Part model, mm, in its own coordinate system. A direction names the side the tool comes from. Coordinates: 2 decimals unless noted, no trailing zeros. Write each loop counter-clockwise with the first axis right and the second up, starting at its lowest first coordinate (ties: lowest second). Pieces come first, ordered by that corner, then holes. Notation, with made-up numbers: (-17.75, -17) - (19.25, -17) arc R31 ccw to (19.25, 14) - close; hole circle Ø6 at (83.25, -27.75). An arc over 180 degrees is marked (long way). Use a Markdown table: item, result.
```python
from build123d import *

# Parameters (mm, degrees)
SKETCH1_W             = 4.084
SKETCH1_H             = 6.24
EXTRUDE1_DEPTH        = 7
SKETCH6_W             = 6.834
SKETCH6_H             = 16.75
EXTRUDE2_DEPTH        = 5.23
F_4_CLEARANCE_HOLE1_D = 3.2
SKETCH3_R             = 1.25
CUT_EXTRUDE1_DEPTH    = 7.24
SKETCH7_W             = 0.217
SKETCH7_H             = 16.75
EXTRUDE3_DEPTH        = 6.23


with BuildPart() as part:
    # Sketch1 → Extrude1 (new body, symmetric)
    with BuildSketch(Plane.XY):
        Rectangle(SKETCH1_W, SKETCH1_H)
    extrude(amount=EXTRUDE1_DEPTH, both=True)

    # Sketch6 → Extrude2 (add)
    with BuildSketch(Plane(origin=(0, 3.12, 0), x_dir=(1, 0, 0), z_dir=(0, 1, 0))):
        Rectangle(SKETCH6_W, SKETCH6_H)
    extrude(amount=-EXTRUDE2_DEPTH)

    # 4 Clearance Hole1 (through all)
    with Locations(Plane(origin=(0.396685659, -3.12, 2.776888518), x_dir=(1, 0, 0), z_dir=(0, -1, 0))):
        with Locations((-0.396685659, -2.776888518)):
            Hole(F_4_CLEARANCE_HOLE1_D / 2)

    # Sketch3 → Cut-Extrude1 (cut, through all)
    with BuildSketch(Plane(origin=(0, -3.12, 0), x_dir=(-1, 0, 0), z_dir=(0, -1, 0))):
        with Locations(Location((0, -5, 0), (0, 0, 180))):  # turned: the seam where the file's is
            Circle(SKETCH3_R)
        with Locations((0, 5)):
            Circle(SKETCH3_R)
    extrude(amount=-CUT_EXTRUDE1_DEPTH, mode=Mode.SUBTRACT)

    # Sketch7 → Extrude3 (cut, through all)
    with BuildSketch(Plane.XZ.offset(2.11)):
        with Locations((3.3085, 0)):
            Rectangle(SKETCH7_W, SKETCH7_H)
    extrude3 = extrude(amount=-EXTRUDE3_DEPTH, mode=Mode.SUBTRACT)

    # Mirror1: Extrude3 across plane
    add(extrude3.mirror(Plane(origin=(0, 0, 0), x_dir=(0, 0, 1), z_dir=(1, 0, 0))), mode=Mode.SUBTRACT)


solid = part.part
```
Item 1: Band-saw the part on B-B, the plane x = 0. Give the cut face in (y, z) (3 decimals), then the cut area to 3 significant figures.
From the geometry:
| item | result |
|---|---|
| outline | (-3.12, -7) - (-2.11, -7) - (-2.11, -8.375) - (3.12, -8.375) - (3.12, -6.25) - (-3.12, -6.25) - close; (-3.12, -3.75) - (3.12, -3.75) - (3.12, -1.6) - (-3.12, -1.6) - close; (-3.12, 1.6) - (3.12, 1.6) - (3.12, 3.75) - (-3.12, 3.75) - close; (-3.12, 6.25) - (3.12, 6.25) - (3.12, 8.375) - (-2.11, 8.375) - (-2.11, 7) - (-3.12, 7) - close |
| area | 50.6 mm^2 |
Item 2: Which spindle directions (+Z, -Z, +X, -X, +Y, -Y) get a long thin tool onto all of the face, cutting with end or side? Do faces 1 (the face through (0, -2.6, -7)), 2 (the face through (2.042, -2.6, 0.1)), 3 (the face through (0, -2.6, 7)). Say none if no direction does.
From the geometry:
| item | result |
|---|---|
| face 1 | -Z, +X, -X, -Y |
| face 2 | +Z, -Z, +X, -Y |
| face 3 | +Z, +X, -X, -Y |
Item 3: Band-saw the part on A-A, the plane z = 0. Give the cut face in (x, y), then the cut area to 3 significant figures.
From the geometry:
| item | result |
|---|---|
| outline | (-3.2, -2.11) - (-2.04, -2.11) - (-2.04, -3.12) - (-1.6, -3.12) - (-1.6, 3.12) - (-3.2, 3.12) - close; (1.6, -3.12) - (2.04, -3.12) - (2.04, -2.11) - (3.2, -2.11) - (3.2, 3.12) - (1.6, 3.12) - close |
| area | 17.6 mm^2 |
Item 4: Band-saw the part on D-D, the plane z = -2.25. Give the cut face in (x, y).
From the geometry:
| item | result |
|---|---|
| outline | (-3.2, -2.11) - (-2.04, -2.11) - (-2.04, -3.12) - (2.04, -3.12) - (2.04, -2.11) - (3.2, -2.11) - (3.2, 3.12) - (-3.2, 3.12) - close |
Item 5: Drill centre lines: probe 1 along Z at (x, y) = (0, -0.5) (3 decimals); probe 2 along X at (y, z) = (0.75, -5); probe 3 along Z at (x, y) = (1, 1.75) (3 decimals). Where is each one in solid material? Low to high.
From the geometry:
| item | result |
|---|---|
| probe 1 | -8.375 to -6.25, -3.75 to -1.6, 1.6 to 3.75, 6.25 to 8.375 |
| probe 2 | -3.2 to -1.25, 1.25 to 3.2 |
| probe 3 | -8.375 to -5.75, -4.25 to -1.249, 1.249 to 4.25, 5.75 to 8.375 |
Item 6: Two-plate mould, pull along Z, no slides. Class faces 4 (the face through (0, 1, 8.375)), 5 (the face through (-0.27, -0.04, 3.78)), 6 (the face through (-2.2, -2.11, -0.1)), 7 (the face through (1.27, 0.04, -0.97)): pulls with the +Z half, pulls with the -Z half, needs draft (parallel to the pull), parting line crosses it, or undercut.
From the geometry:
| item | result |
|---|---|
| face 4 | pulls with the +Z half |
| face 5 | undercut |
| face 6 | needs draft |
| face 7 | undercut |
Item 7: Band-saw the part on C-C, the plane y = 2.5. Give the cut face in (x, z) (3 decimals), then the cut area to 3 significant figures.
From the geometry:
| item | result |
|---|---|
| outline | (-3.2, -8.375) - (3.2, -8.375) - (3.2, 8.375) - (-3.2, 8.375) - close; hole circle Ø3.2 at (0, 0); hole circle Ø2.5 at (0, -5); hole circle Ø2.5 at (0, 5) |
| area | 89.3 mm^2 |
Item 8: Drop flat-ended pins along their axis: P1, Ø1.1, axis at y = -2.5, z = 1, coming from the -X side; P2, Ø0.5, axis at y = -2.5, z = -2.5, coming from the +X side. Give the stop position or say it passes through.
From the geometry:
| item | result |
|---|---|
| P1 | x = -3.2 |
| P2 | x = 2.04 |
